Check sheet for the modelled part. Datum: model origin and axes. Units: mm. A direction names the side the tool comes from. Coordinates: 2 decimals unless noted, no trailing zeros. Write each loop counter-clockwise with the first axis right and the second up, starting at its lowest first coordinate (ties: lowest second). Pieces come first, ordered by that corner, then holes. Notation, with made-up numbers: M -12,54.25 L 37,54.25 A28 cw 37,92.25 Z; hole C 40,-12 d11. An arc over 180 degrees is marked long. Answer as CSV lines item,"result". Start each with the question number.
1) Section check C-C (x = 158.5). Record the cut outline in (y, z).
2) Section check A-A (z = -15). State how many separate pieces and enclosed holes the cut face has, and give its area (3 significant figures).
3) Go/stop test with flat-tipped pins: pin 1 Ø0.9 at (y, z) = (15, -13.5) entering from -X; pin 2 Ø1.5 at (x, z) = (114, -27) entering from +Y. Record where each tip stops, or that it passes through.
4) Material ranges on L1, parallel to X at y = -2, z = -28.5; L2, parallel to Y at x = 158, z = -26.75; L3, parallel to X at y = 2, z = -15, recorded low to high. Write a range as [from, to].
5) Section check D-D (x = 41). Record the cut outline in (y, z), and give its area (3 significant figures).
6) Draft check along Z on faces 4 (the flat face through (102.5, -3, -5)), 5 (the flat face through (98, -3, -10)). Enter one of: +Z half, -Z half, draft (parallel to the pull), parting line (faces both ways), or undercut.
7) Access from +Z, -Z, +X, -X, +Y, -Y to the whole of each face (thin tool, end or side, straight path). Record for faces 1 (the flat face through (92.5, -3, -5)), 2 (the cylindrical face through (191.553, 13.098, -3.451)), 3 (the cylindrical face through (129, 19, -27)).
8) Section check B-B (x = 83.2). Record the cut outline in (y, z).
from build123d import *

# Parameters (mm, degrees)
SKETCH1_W           = 195
SKETCH1_H           = 30
BOSS_EXTRUDE1_DEPTH = 8
SKETCH2_W           = 12
SKETCH2_H           = 30
BOSS_EXTRUDE2_DEPTH = 12
SKETCH4_R           = 3.15
CUT_EXTRUDE1_DEPTH  = 199.305320151
FILLET1_R           = 4
FILLET2_R           = 6
BOSS_EXTRUDE4_DEPTH = 30
SKETCH15_W          = 67
SKETCH15_H          = 7
BOSS_EXTRUDE6_DEPTH = 13
SKETCH16_W          = 62
SKETCH16_H          = 6.3
CUT_EXTRUDE4_DEPTH  = 199.408669165
FILLET6_R           = 5
FILLET7_R           = 5
SKETCH17_W          = 10
SKETCH17_H          = 30
BOSS_EXTRUDE7_DEPTH = 6
FILLET8_R           = 3.15
FILLET9_R           = 5
SKETCH20_R          = 3.15
BOSS_EXTRUDE8_DEPTH = 16
SKETCH21_W          = 10
SKETCH21_H          = 30
BOSS_EXTRUDE9_DEPTH = 6
SKETCH22_W          = 10
SKETCH22_H          = 10
CUT_EXTRUDE5_DEPTH  = 6
FILLET10_R          = 5
FILLET11_R          = 3.15
SKETCH23_R          = 3.25
CUT_EXTRUDE6_DEPTH  = 199.408669165


with BuildPart() as part:
    # Sketch1 → Boss-Extrude1 (new body)
    with BuildSketch(Plane(origin=(0, 0, 0), x_dir=(1, 0, 0), z_dir=(0, 1, 0))):
        with Locations((97.5, 15)):
            Rectangle(SKETCH1_W, SKETCH1_H)
    extrude(amount=BOSS_EXTRUDE1_DEPTH)

    # Sketch2 → Boss-Extrude2 (add)
    with BuildSketch(Plane(origin=(0, 8, 0), x_dir=(1, 0, 0), z_dir=(0, 1, 0))):
        with Locations((10.715252385, 15)):
            Rectangle(SKETCH2_W, SKETCH2_H)
    extrude(amount=BOSS_EXTRUDE2_DEPTH)

    # Sketch4 → Cut-Extrude1 (cut, through all)
    with BuildSketch(Plane(origin=(0, 0, -30), x_dir=(-1, 0, 0), z_dir=(0, 0, -1))):
        with Locations((-10.715252385, 14)):
            Circle(SKETCH4_R)
    extrude(amount=-CUT_EXTRUDE1_DEPTH, mode=Mode.SUBTRACT)

    # Fillet1
    fillet1_edges = [part.edges().sort_by_distance(p)[0] for p in [
        (4.715252385, 8, -15),
        (16.715252385, 8, -15),
    ]]
    fillet(fillet1_edges, radius=FILLET1_R)

    # Fillet2
    fillet2_edges = [part.edges().sort_by_distance(p)[0] for p in [
        (4.715252385, 20, -15),
        (16.715252385, 20, -15),
    ]]
    fillet(fillet2_edges, radius=FILLET2_R - 0.0001)  # a hair under: the kernel refuses the full size

    # Sketch11 → Boss-Extrude4 (add)
    with BuildSketch(Plane(origin=(0, 0, -30), x_dir=(-1, 0, 0), z_dir=(0, 0, -1))):
        with BuildLine():
            Line((-16.715252385, 14), (-16.715252385, 12))
            ThreePointArc((-16.715252385, 12), (-17.88682526, 9.171572875), (-20.715252385, 8))
            Line((-20.715252385, 8), (-22.27876013, 8))
            Line((-22.27876013, 8), (-20.715252385, 9))
            ThreePointArc((-20.715252385, 9), (-18.593932042, 9.878679656), (-17.715252385, 12))
            Line((-17.715252385, 12), (-17.715252385, 14))
            ThreePointArc((-17.715252385, 14), (-15.664999853, 18.949747468), (-10.715252385, 21))
            ThreePointArc((-10.715252385, 21), (-5.765504917, 18.949747468), (-3.715252385, 14))
            Line((-3.715252385, 14), (-3.715252385, 12))
            ThreePointArc((-3.715252385, 12), (-2.836572729, 9.878679656), (-0.715252385, 9))
            Line((-0.715252385, 9), (0, 8))
            Line((0, 8), (-0.715252385, 8))
            ThreePointArc((-0.715252385, 8), (-3.54367951, 9.171572875), (-4.715252385, 12))
            Line((-4.715252385, 12), (-4.715252385, 14))
            ThreePointArc((-4.715252385, 14), (-6.472611698, 18.242640687), (-10.715252385, 20))
            ThreePointArc((-10.715252385, 20), (-14.957893072, 18.242640687), (-16.715252385, 14))
        make_face()
    extrude(amount=-BOSS_EXTRUDE4_DEPTH)

    # Sketch15 → Boss-Extrude6 (add)
    with BuildSketch(Plane(origin=(0, 8, 0), x_dir=(1, 0, 0), z_dir=(0, 1, 0))):
        with Locations((161.5, 26.5)):
            Rectangle(SKETCH15_W, SKETCH15_H)
        with Locations((161.5, 3.5)):
            Rectangle(SKETCH15_W, SKETCH15_H)
    extrude(amount=BOSS_EXTRUDE6_DEPTH)

    # Sketch16 → Cut-Extrude4 (cut, through all)
    with BuildSketch(Plane(origin=(0, 0, -30), x_dir=(-1, 0, 0), z_dir=(0, 0, -1))):
        with Locations((-161.5, 15.35)):
            Rectangle(SKETCH16_W, SKETCH16_H)
    extrude(amount=-CUT_EXTRUDE4_DEPTH, mode=Mode.SUBTRACT)

    # Fillet6
    fillet6_edges = [part.edges().sort_by_distance(p)[0] for p in [
        (195, 21, -26.5),
        (128, 21, -26.5),
    ]]
    fillet(fillet6_edges, radius=FILLET6_R)

    # Fillet7
    fillet7_edges = [part.edges().sort_by_distance(p)[0] for p in [
        (128, 8, -26.5),
    ]]
    fillet(fillet7_edges, radius=FILLET7_R)

    # Sketch17 → Boss-Extrude7 (add)
    with BuildSketch(Plane.XZ):
        with Locations((97.5, -15)):
            Rectangle(SKETCH17_W, SKETCH17_H)
    extrude(amount=BOSS_EXTRUDE7_DEPTH)

    # Fillet8
    fillet8_edges = [part.edges().sort_by_distance(p)[0] for p in [
        (192.5, 18.5, -3.5),
        (192.5, 12.2, -3.5),
        (130.5, 18.5, -3.5),
        (130.5, 12.2, -3.5),
    ]]
    fillet(fillet8_edges, radius=FILLET8_R - 0.0001)  # a hair under: the kernel refuses the full size

    # Fillet9
    fillet9_edges = [part.edges().sort_by_distance(p)[0] for p in [
        (128, 8, -3.5),
    ]]
    fillet(fillet9_edges, radius=FILLET9_R)

    # Sketch20 → Boss-Extrude8 (add)
    with BuildSketch(Plane.XY.offset(-23)):
        with BuildLine():
            Line((195, 0), (195, 21))
            Line((195, 21), (128, 21))
            Line((128, 21), (128, 13))
            ThreePointArc((128, 13), (126.535533906, 9.464466094), (123, 8))
            Line((123, 8), (22.27876013, 8))
            Line((22.27876013, 8), (20.715252385, 9))
            ThreePointArc((20.715252385, 9), (18.593932042, 9.878679656), (17.715252385, 12))
            Line((17.715252385, 12), (17.715252385, 14))
            ThreePointArc((17.715252385, 14), (10.715252385, 21), (3.715252385, 14))
            Line((3.715252385, 14), (3.715252385, 12))
            ThreePointArc((3.715252385, 12), (2.836572729, 9.878679656), (0.715252385, 9))
            Line((0.715252385, 9), (0, 8))
            Line((0, 8), (0, 0))
            Line((0, 0), (92.5, 0))
            Line((92.5, 0), (92.5, -6))
            Line((92.5, -6), (102.5, -6))
            Line((102.5, -6), (102.5, 0))
            Line((102.5, 0), (195, 0))
        make_face()
        with Locations(Location((10.715252385, 14, 0), (0, 0, 180))):
            Circle(SKETCH20_R, mode=Mode.SUBTRACT)
        with BuildLine():
            Line((133.65, 12.2), (189.35, 12.2))
            ThreePointArc((189.35, 12.2), (191.577386361, 13.122613639), (192.5, 15.35))
            ThreePointArc((192.5, 15.35), (191.577386361, 17.577386361), (189.35, 18.5))
            Line((189.35, 18.5), (133.65, 18.5))
            ThreePointArc((133.65, 18.5), (131.422613639, 17.577386361), (130.5, 15.35))
            ThreePointArc((130.5, 15.35), (131.422613639, 13.122613639), (133.65, 12.2))
        make_face(mode=Mode.SUBTRACT)
    extrude(amount=BOSS_EXTRUDE8_DEPTH)

    # Sketch21 → Boss-Extrude9 (add)
    with BuildSketch(Plane(origin=(0, 0, 0), x_dir=(-1, 0, 0), z_dir=(0, -1, 0))):
        with Locations((-5, 15)):
            Rectangle(SKETCH21_W, SKETCH21_H)
        with Locations((-190, 15)):
            Rectangle(SKETCH21_W, SKETCH21_H)
    extrude(amount=BOSS_EXTRUDE9_DEPTH)

    # Sketch22 → Cut-Extrude5 (cut)
    with BuildSketch(Plane(origin=(0, -6, 0), x_dir=(-1, 0, 0), z_dir=(0, -1, 0))):
        with Locations((-5, 15)):
            Rectangle(SKETCH22_W, SKETCH22_H)
        with Locations((-97.5, 15)):
            Rectangle(SKETCH22_W, SKETCH22_H)
        with Locations((-190, 15)):
            Rectangle(SKETCH22_W, SKETCH22_H)
    extrude(amount=-CUT_EXTRUDE5_DEPTH, mode=Mode.SUBTRACT)

    # Fillet10
    fillet10_edges = [part.edges().sort_by_distance(p)[0] for p in [
        (128, 21, -11.5),
        (195, 21, -11.5),
    ]]
    fillet(fillet10_edges, radius=FILLET10_R)

    # Fillet11
    fillet11_edges = [part.edges().sort_by_distance(p)[0] for p in [
        (130.5, 18.5, -26.5),
        (130.5, 12.2, -26.5),
        (192.5, 12.2, -26.5),
        (192.5, 18.5, -26.5),
    ]]
    fillet(fillet11_edges, radius=FILLET11_R - 0.0001)  # a hair under: the kernel refuses the full size

    # Sketch23 → Cut-Extrude6 (cut, through all)
    with BuildSketch(Plane.XZ):
        with Locations(Location((83.2, -15, 0), (0, 0, 270))):
            Circle(SKETCH23_R)
        with Locations(Location((111.8, -15, 0), (0, 0, 270))):
            Circle(SKETCH23_R)
    extrude(amount=-CUT_EXTRUDE6_DEPTH, mode=Mode.SUBTRACT)


solid = part.part
Results found:
1,outline,"M 0,-30 L 12.2,-30 L 12.2,0 L 0,0 Z; M 18.5,-30 L 21,-30 L 21,0 L 18.5,0 Z"
2,separate pieces,"3"
2,enclosed holes,"2"
2,area,"2,080 mm2"
3,pin 1,"stops at x = 3.74"
3,pin 2,"stops at y = 8"
4,L1,"x = [0, 10], [92.5, 102.5], [185, 195]"
4,L2,"y = [0, 12.2], [18.5, 21]"
4,L3,"x = [0, 79.95], [86.45, 108.55], [115.05, 195]"
5,outline,"M 0,-30 L 8,-30 L 8,0 L 0,0 Z"
5,area,"240 mm2"
6,face 4,"draft"
6,face 5,"undercut"
7,face 1,"+Z, -Z, -Y"
7,face 2,"+Z, -Z"
7,face 3,"+Z, -Z, +Y"
8,outline,"M 0,-30 L 8,-30 L 8,-18.25 L 0,-18.25 Z; M 0,-11.75 L 8,-11.75 L 8,0 L 0,0 Z"
